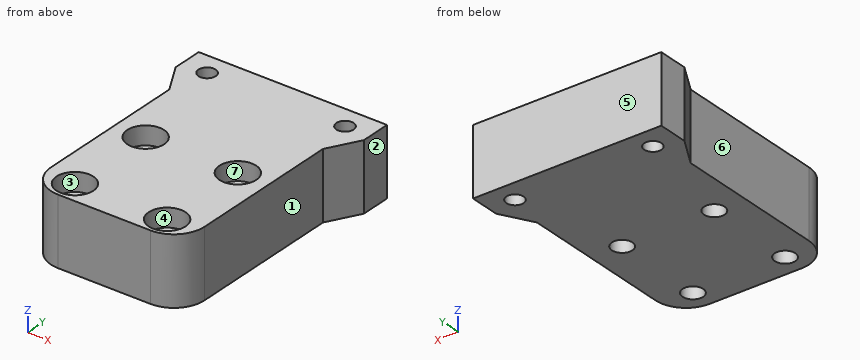
```python
from build123d import *

# Parameters (mm, degrees)
F0_W     = 25
F0_H     = 30.0927665085
F0_W_2   = 30.6387297809
F0_H_2   = 4.8959264159
F1_DEPTH = 11
F2_R     = 1.675
F3_DEPTH = 25
F4_R     = 5
F5_DEPTH = 11
F6_R     = 1.4
F7_DEPTH = 11.001
F2_R_2   = 3
F8_DEPTH = 3


# Not quite as in the source:
# - a feature names something its author has since deleted; it is built from what else it names


with BuildPart() as f1:
    # F0 (on Top) → F1 (new body)
    with BuildSketch(Plane.XY):
        with Locations((12.5, 15.0463832542)):
            Rectangle(F0_W, F0_H)
        Polygon((-2.8193648905, 35.1040735841), (0, 30.0927665085), (25, 30.0927665085), (27.8193648905, 35.1040735841), align=None)
        with Locations((12.5, 37.552036792)):
            Rectangle(F0_W_2, F0_H_2)
    extrude(amount=F1_DEPTH)

    # F2 (on face) → F3 (cut)
    with BuildSketch(Plane.XY.offset(11)):
        with BuildLine():
            ThreePointArc((3.325, 18.5605346784), (5, 16.8855346784), (6.675, 18.5605346784))
            ThreePointArc((6.675, 18.5605346784), (5, 20.2355346784), (3.325, 18.5605346784))
        make_face()
        with Locations((20, 18.5605346784)):
            Circle(F2_R)
        with Locations((20, 3.5605346784)):
            Circle(F2_R)
        with Locations((5, 3.5605346784)):
            Circle(F2_R)
    extrude(amount=-F3_DEPTH, mode=Mode.SUBTRACT)

    # F4
    f4_edges = [f1.edges().sort_by_distance(p)[0] for p in [
        (0, 0, 5.5),
        (25, 0, 5.5),
    ]]
    fillet(f4_edges, radius=F4_R)

    # F0 (on Top) → F5 (join)
    with BuildSketch(Plane.XY):
        with Locations((12.5, 37.552036792)):
            Rectangle(F0_W_2, F0_H_2)
        Polygon((-2.8193648905, 35.1040735841), (0, 30.0927665085), (25, 30.0927665085), (27.8193648905, 35.1040735841), align=None)
    extrude(amount=F5_DEPTH)

    # F6 (on face) → F7 (cut, through all)
    with BuildSketch(Plane.XY.offset(11)):
        with Locations((23.7225, 36.4378243685)):
            Circle(F6_R)
        with BuildLine():
            ThreePointArc((-0.1225, 36.4378243685), (1.2775, 35.0378243685), (2.6775, 36.4378243685))
            ThreePointArc((2.6775, 36.4378243685), (1.2775, 37.8378243685), (-0.1225, 36.4378243685))
        make_face()
    extrude(amount=-F7_DEPTH, mode=Mode.SUBTRACT)

    # F2 (on face) → F8 (cut)
    with BuildSketch(Plane.XY.offset(11)):
        with BuildLine():
            ThreePointArc((8, 18.5605346784), (5, 21.5605346784), (2, 18.5605346784))
            ThreePointArc((2, 18.5605346784), (5, 15.5605346784), (8, 18.5605346784))
        make_face()
        with BuildLine():
            ThreePointArc((3.325, 18.5605346784), (5, 20.2355346784), (6.675, 18.5605346784))
            ThreePointArc((6.675, 18.5605346784), (5, 16.8855346784), (3.325, 18.5605346784))
        make_face(mode=Mode.SUBTRACT)
        with Locations((5, 3.5605346784)):
            Circle(F2_R_2)
        with Locations((5, 3.5605346784)):
            Circle(F2_R, mode=Mode.SUBTRACT)
        with Locations((20, 18.5605346784)):
            Circle(F2_R_2)
        with Locations((20, 18.5605346784)):
            Circle(F2_R, mode=Mode.SUBTRACT)
        with Locations((20, 3.5605346784)):
            Circle(F2_R_2)
        with Locations((20, 3.5605346784)):
            Circle(F2_R, mode=Mode.SUBTRACT)
    extrude(amount=-F8_DEPTH, mode=Mode.SUBTRACT)


solid = f1.part
```
Input: part model. Units: mm. Frame: model coordinates. Face numbers are marked on the shaded views. A direction names the side the tool comes from. Round coordinates to 2 decimals unless told otherwise and drop trailing zeros. Loops run counter-clockwise (first coordinate to the right, second up) from the corner with the lowest first, then second, coordinate; pieces in that order, holes last. Notation, with made-up numbers: M 53,46.25 L 93,46.25 A13 cw 93,59.25 Z; hole C 71,67 d2. An arc over 180 degrees is marked long. Answer in a Markdown table with one row per item. Add a question column.
1. Section B-B (y = 17.5). Output: boundary loops of the cut face in (x, z), and give its area (3 significant figures).
2. Contact query for flat-ended pins moving along their axis: pin 1 (1 mm diameter, centred on y = 6.5, z = 10, fed in from -X); pin 2 (1.8 mm diameter, centred on x = 6, y = 17.5, fed in from +Z); pin 3 (2 mm diameter, centred on y = 24, z = 5.5, fed in from +X). Output: stop coordinate, or through.
3. Section D-D (y = 11). Output: boundary loops of the cut face in (x, z), and give its area (3 significant figures).
4. Section A-A (x = 19). Output: boundary loops of the cut face in (y, z).
5. Ray query, probe 1 along Y at (x, z) = (5, 2.75); probe 2 along Y at (x, z) = (20, 9.95); probe 3 along X at (y, z) = (36, 3.5). Return the intervals inside material, ascending.
6. Section C-C (z = 9.5). Output: boundary loops of the cut face in (x, y).
7. Mould query, pull axis X, two halves, no side actions, for the marked faces 4, 5, 6 and 7. Classes: released by +X, released by -X, zero draft, split by the parting line, or undercut.
8. Set-up query: the marked faces 1, 2 and 3. Return all of +Z, -Z, +X, -X, +Y, -Y with unobstructed straight access to the full face (end or side cutting, diameter ignored); none if empty.
Values follow:
| question | item | result |
|---|---|---|
| 1 | outline | M 0,0 L 3.7,0 L 3.7,8 L 2.19,8 L 2.19,11 L 0,11 Z; M 6.3,0 L 18.7,0 L 18.7,8 L 17.19,8 L 17.19,11 L 7.81,11 L 7.81,8 L 6.3,8 Z; M 21.3,0 L 25,0 L 25,11 L 22.81,11 L 22.81,8 L 21.3,8 Z |
| 1 | area | 200 mm^2 |
| 2 | pin 1 | x = 0 |
| 2 | pin 2 | z = 8 |
| 2 | pin 3 | x = 25 |
| 3 | outline | M 0,0 L 25,0 L 25,11 L 0,11 Z |
| 3 | area | 275 mm^2 |
| 4 | outline | M 0,0 L 2.22,0 L 2.22,8 L 0.73,8 L 0.73,11 L 0,11 Z; M 4.9,0 L 17.22,0 L 17.22,8 L 15.73,8 L 15.73,11 L 6.39,11 L 6.39,8 L 4.9,8 Z; M 19.9,0 L 40,0 L 40,11 L 21.39,11 L 21.39,8 L 19.9,8 Z |
| 5 | probe 1 | 0 to 1.89, 5.24 to 16.89, 20.24 to 40 |
| 5 | probe 2 | 0 to 0.56, 6.56 to 15.56, 21.56 to 40 |
| 5 | probe 3 | -2.82 to -0.05, 2.61 to 22.39, 25.05 to 27.82 |
| 6 | outline | M -2.82,35.1 L 0,30.09 L 0,5 A5 ccw 5,0 L 20,0 A5 ccw 25,5 L 25,30.09 L 27.82,35.1 L 27.82,40 L -2.82,40 Z; hole C 1.28,36.44 d2.8; hole C 5,3.56 d6; hole C 5,18.56 d6; hole C 20,3.56 d6; hole C 20,18.56 d6; hole C 23.72,36.44 d2.8 |
| 7 | face 4 | undercut |
| 7 | face 5 | zero draft |
| 7 | face 6 | released by -X |
| 7 | face 7 | undercut |
| 8 | face 1 | +Z, -Z, +X, -Y |
| 8 | face 2 | +Z, -Z, +X, +Y, -Y |
| 8 | face 3 | +Z |
